from build123d import *

# Parameters (mm, degrees)
F1_DEPTH = 3.175


with BuildPart() as f1:
    # F0 (on Front) → F1 (new body, symmetric)
    with BuildSketch(Plane.XZ):
        Polygon((21.252101, -4.937558), (180.730679, -97.012558), (183.905679, -91.513296), (18.927839, 3.736704), align=None)
        Polygon((12.577839, -7.261819), (177.555679, -102.511819), (180.730679, -97.012558), (21.252101, -4.937558), align=None)
        Polygon((180.730679, -97.012558), (186.22994, -100.187558), (183.905679, -91.513296), align=None)
        Polygon((180.730679, -97.012558), (177.555679, -102.511819), (186.22994, -100.187558), align=None)
    extrude(amount=F1_DEPTH, both=True)


solid = f1.part
Geometry check sheet. Reference: the model listing, model coordinates, mm. A direction names the side the tool comes from. Round coordinates to 2 decimals unless told otherwise and drop trailing zeros. Loops run counter-clockwise (first coordinate to the right, second up) from the corner with the lowest first, then second, coordinate; pieces in that order, holes last.
Item 1: Cross-section at A-A on y = -0.5. Record the boundary of the cut face in (x, z).
Item 2: Gauge pin test, flat ends, axial feed: pin 1 (1.5 mm diameter, centred on y = -1, z = -34, fed in from -X); pin 2 (2 mm diameter, centred on x = 143, y = 1.5, fed in from +Z); pin 3 (1 mm diameter, centred on x = 115, y = -1.5, fed in from -Z). Record the tip position at first contact, or that the pin passes through.
Item 3: Cross-section at C-C on z = -25. Record the boundary of the cut face in (x, y) (3 decimals).
Item 4: Cross-section at B-B on x = 58. Record the boundary of the cut face in (y, z) (3 decimals).
Item 5: Access from +Z, -Z, +X, -X, +Y, -Y to the whole of each face (thin tool, end or side, straight path). Record for faces 4 (the flat face through (185.084, -0.044, -95.911)), 5 (the flat face through (20.074, -0.044, -0.54)).
Item 6: Thickness scan on line 1 (Z direction, x = 152, y = -0.75); line 2 (Z direction, x = 146.5, y = -1.25); line 3 (X direction, y = 0, z = -48.5). Record the ranges inside material, lowest first.
Item 7: Mould release check, pull along Z, two halves, no side actions. Record for faces 1 (the flat face through (99, 3.175, -49)), 2 (the flat face through (16.976, -0.044, -6.083)), 3 (the flat face through (102.572, -0.044, -44.555)): pulls with the +Z half, pulls with the -Z half, needs draft (parallel to the pull), parting line crosses it, or undercut.
Answer sheet:
1. outline: (12.58, -7.26) - (177.56, -102.51) - (186.23, -100.19) - (183.91, -91.51) - (18.93, 3.74) - (21.25, -4.94) - close
2. pin 1: stops at x = 57.59
2. pin 2: stops at z = -67.32
2. pin 3: stops at z = -66.68
3. outline: (43.301, -3.175) - (68.701, -3.175) - (68.701, 3.175) - (43.301, 3.175) - close
4. outline: (-3.175, -33.486) - (3.175, -33.486) - (3.175, -18.822) - (-3.175, -18.822) - close
5. face 4: +Z, +X, +Y, -Y
5. face 5: -X, +Y, -Y
6. line 1: z = -87.76 to -73.09
6. line 2: z = -84.58 to -69.92
6. line 3: x = 84 to 109.4
7. face 1: needs draft
7. face 2: undercut
7. face 3: pulls with the +Z half
